Can you work these out from the model? Positions are in its coordinate system, mm. Face numbers are marked on the shaded views. A direction names the side the tool comes from. Coordinates: 2 decimals unless noted, no trailing zeros. Loops run counter-clockwise (first coordinate to the right, second up) from the corner with the lowest first, then second, coordinate; pieces in that order, holes last. Notation, with made-up numbers: M 49.5,-10.5 L 100.5,-10.5 A10 ccw 100.5,-3.5 Z; hole C 80.5,43 d4. An arc over 180 degrees is marked long. Return JSON: item names as keys, results as strings. Group by question number.
```python
from build123d import *

# Parameters (mm, degrees)
SKETCH1_W           = 79
SKETCH1_H           = 50.8
SKETCH1_R           = 2.1
BOSS_EXTRUDE1_DEPTH = 6
SKETCH3_W           = 15
SKETCH3_H           = 50.8
BOSS_EXTRUDE2_DEPTH = 15


with BuildPart() as part:
    # Sketch1 → Boss-Extrude1 (new body)
    with BuildSketch(Plane.XY):
        with Locations((39.5, 25.4)):
            Rectangle(SKETCH1_W, SKETCH1_H)
        with Locations((67, 39.4)):
            Circle(SKETCH1_R, mode=Mode.SUBTRACT)
        with Locations((67, 11.4)):
            Circle(SKETCH1_R, mode=Mode.SUBTRACT)
        with Locations((39, 39.4)):
            Circle(SKETCH1_R, mode=Mode.SUBTRACT)
        with Locations((39, 11.4)):
            Circle(SKETCH1_R, mode=Mode.SUBTRACT)
    extrude(amount=BOSS_EXTRUDE1_DEPTH)

    # Sketch3 → Boss-Extrude2 (add)
    with BuildSketch(Plane(origin=(0, 0, 0), x_dir=(-1, 0, 0), z_dir=(0, 0, -1))):
        with Locations((-7.5, 25.4)):
            Rectangle(SKETCH3_W, SKETCH3_H)
    extrude(amount=BOSS_EXTRUDE2_DEPTH)


solid = part.part
```
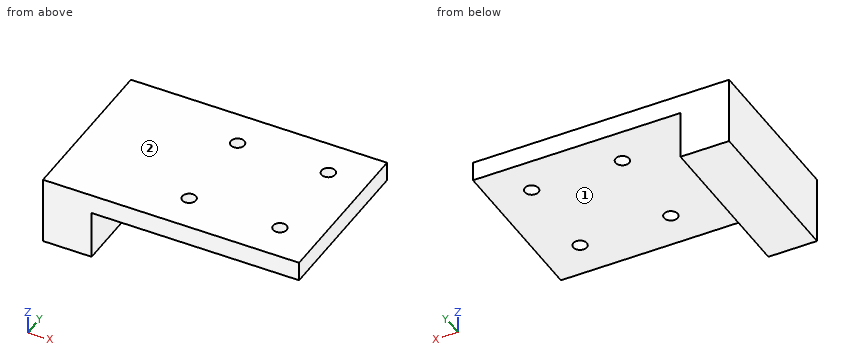
1) Suppose I cut it at C-C, the plane x = 49. List the corners of the cut face in (y, z) for me, then the cut area to 3 significant figures.
2) Suppose I cut it at A-A, the plane y = 39.4. List the corners of the cut face in (x, z) for me, then the cut area to 3 significant figures.
3) For the marked faces 1 and 2, which set-ups out of +Z, -Z, +X, -X, +Y, -Y let a thin tool reach every point of the face, with its end or its side?
4) Suppose I cut it at B-B, the plane x = 39. List the corners of the cut face in (y, z) for me, then the cut area to 3 significant figures.
5) For pin 1 (12 mm diameter, centred on x = 29.5, y = 40.5, fed in from -Z); pin 2 (4.5 mm diameter, centred on y = 13, z = -7, fed in from +X), each with a flat end and sliding along its axis, tell me the tip position at first contact or that it passes through.
6) Suppose I cut it at D-D, the plane z = -9.75. List the corners of the cut face in (x, y) for me.
7) If I drill on line 1 (Y direction, x = 67, z = 1.65); line 2 (X direction, y = 47, z = -9.75); line 3 (Z direction, x = 60, y = 30), over which ranges is the centre line in solid material (lowest first)? Write a range as from..to.
Returned:
{
 "1": {"outline": "M 0,0 L 50.8,0 L 50.8,6 L 0,6 Z", "area": "305 mm²"},
 "2": {"outline": "M 0,-15 L 15,-15 L 15,0 L 36.9,0 L 36.9,6 L 0,6 Z; M 41.1,0 L 64.9,0 L 64.9,6 L 41.1,6 Z; M 69.1,0 L 79,0 L 79,6 L 69.1,6 Z", "area": "649 mm²"},
 "3": {"face 1": "-Z, +X, +Y, -Y", "face 2": "+Z, +X, -X, +Y, -Y"},
 "4": {"outline": "M 0,0 L 9.3,0 L 9.3,6 L 0,6 Z; M 13.5,0 L 37.3,0 L 37.3,6 L 13.5,6 Z; M 41.5,0 L 50.8,0 L 50.8,6 L 41.5,6 Z", "area": "254 mm²"},
 "5": {"pin 1": "stops at z = 0", "pin 2": "stops at x = 15"},
 "6": {"outline": "M 0,0 L 15,0 L 15,50.8 L 0,50.8 Z"},
 "7": {"line 1": "y = 0..9.3, 13.5..37.3, 41.5..50.8", "line 2": "x = 0..15", "line 3": "z = 0..6"}
}
